Answer from the drawing. Dimensions are ordinates in mm from the lowest x, y and z of the part. A direction names the side the tool comes from. Coordinates: 2 decimals unless noted, no trailing zeros. Loops run counter-clockwise (first coordinate to the right, second up) from the corner with the lowest first, then second, coordinate; pieces in that order, holes last. Notation, with made-up numbers: (57, 32.5) - (68, 32.5) arc R24 ccw to (68, 63.5) - close; hole circle Ø7 at (4, 82.25). An arc over 180 degrees is marked (long way). Use one line per item in the form item = value. Start each with the question number.
1) Which of the six approach directions +Z, -Z, +X, -X, +Y, -Y give full straight-line access (tool end or side, diameter ignored) to the marked faces 4, 5 and 6?
2) Each of these flat-tipped pins is pushed along its axis until it touches: P1, Ø3, axis at x = 3, y = 6.5, coming from the -Z side; P2, Ø5, axis at x = 7.5, z = 58.5, coming from the +Y side; P3, Ø5, axis at x = 5, z = 26, coming from the -Y side. Where does it stop, or does it pass through?
3) The mould has two halves that part along Z. Classify the marked faces 1, 2 and 3: released by +Z, released by -Z, zero draft, split by the parting line, or undercut.
4) A cutting plane is placed at D-D (z = 61). Give the vertices of the cut face in (x, y), and give its area (3 significant figures).
5) Consider line 1 (Z direction, x = 3, y = 56.5); line 2 (Y direction, x = 4.75, z = 91); line 3 (Y direction, x = 1.75, z = 63). Determine where each line is inside the solid, lowest interval first.
6) A cutting plane is placed at C-C (z = 30.5). Give the vertices of the cut face in (x, y).
7) A cutting plane is placed at B-B (x = 6.25). Give the vertices of the cut face in (y, z).
8) A cutting plane is placed at A-A (y = 51). Give the vertices of the cut face in (x, z).
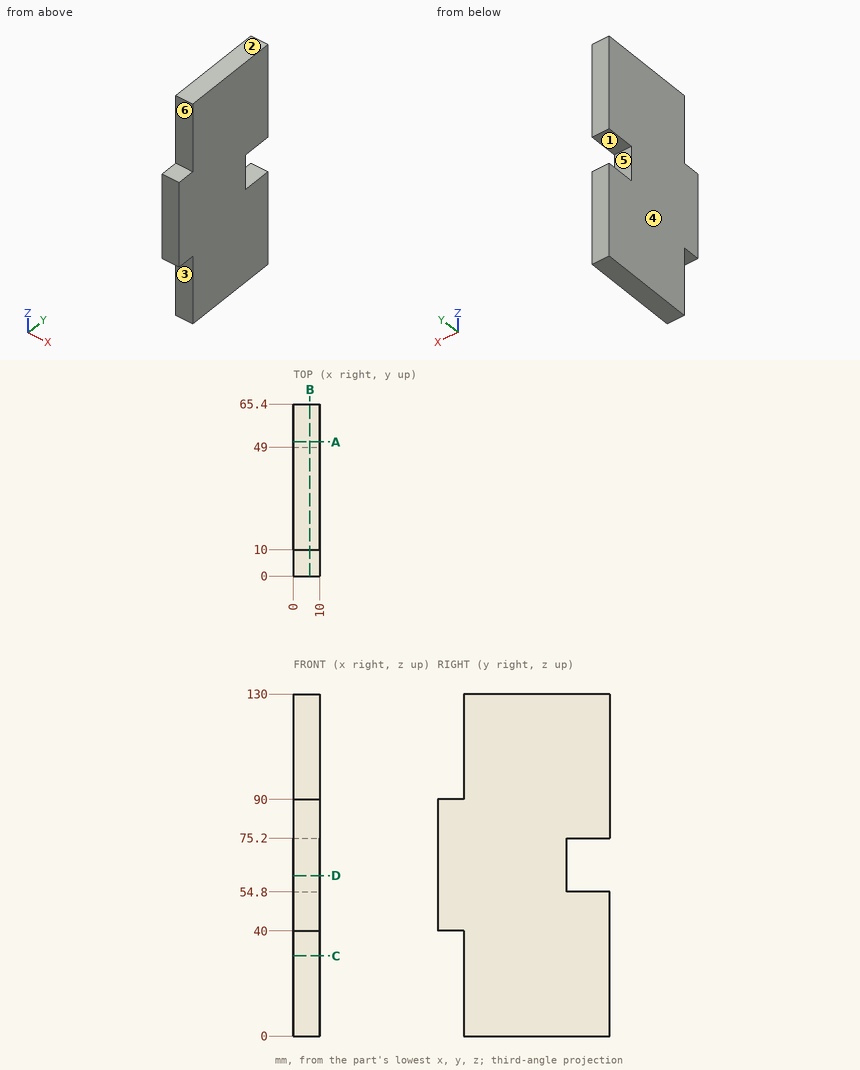
Found:
q1.face_4 = +Z, -Z, -X, +Y, -Y
q1.face_5 = +X, -X, +Y
q1.face_6 = +Z, +X, -X, -Y
q2.P1 = 40
q2.P2 = 49
q2.P3 = 10
q3.face_1 = undercut
q3.face_2 = released by +Z
q3.face_3 = zero draft
q4.outline = (0, 0) - (10, 0) - (10, 49) - (0, 49) - close
q4.area = 490 mm^2
q5.line_1 = 0 to 54.8, 75.2 to 130
q5.line_2 = 10 to 65.4
q5.line_3 = 0 to 49
q6.outline = (0, 10) - (10, 10) - (10, 65.4) - (0, 65.4) - close
q7.outline = (0, 40) - (10, 40) - (10, 0) - (65.4, 0) - (65.4, 54.8) - (49, 54.8) - (49, 75.2) - (65.4, 75.2) - (65.4, 130) - (10, 130) - (10, 90) - (0, 90) - close
q8.outline = (0, 0) - (10, 0) - (10, 54.8) - (0, 54.8) - close; (0, 75.2) - (10, 75.2) - (10, 130) - (0, 130) - close
